```python
from build123d import *

# Parameters (mm, degrees)
ESQUISSE1_W             = 50
ESQUISSE1_H             = 80
BOSS_EXTRU_1_DEPTH      = 2
ENL_V_MAT_EXTRU_1_REACH = 4
ESQUISSE2_R             = 1.75


with BuildPart() as part:
    # Esquisse1 → Boss.-Extru.1 (new body)
    with BuildSketch(Plane(origin=(0, 0, 0), x_dir=(1, 0, 0), z_dir=(0, 1, 0))):
        with Locations((25, 40)):
            Rectangle(ESQUISSE1_W, ESQUISSE1_H)
    extrude(amount=BOSS_EXTRU_1_DEPTH)

    # Esquisse2 → Enlèv. mat.-Extru.1 (cut, up to next)
    with BuildSketch(Plane(origin=(0, 2, 0), x_dir=(1, 0, 0), z_dir=(0, 1, 0)), mode=Mode.PRIVATE) as enl_v_mat_extru_1_sk1:
        with Locations((12.5, 56)):
            Circle(ESQUISSE2_R)
    enl_v_mat_extru_1_tool1 = extrude(enl_v_mat_extru_1_sk1.sketch, amount=-ENL_V_MAT_EXTRU_1_REACH, mode=Mode.PRIVATE) & part.part
    add(enl_v_mat_extru_1_tool1.solids().sort_by_distance((12.5, 2, -56))[0], mode=Mode.SUBTRACT)
    # Esquisse2 → Enlèv. mat.-Extru.1 (cut, up to next)
    with BuildSketch(Plane(origin=(0, 2, 0), x_dir=(1, 0, 0), z_dir=(0, 1, 0)), mode=Mode.PRIVATE) as enl_v_mat_extru_1_sk2:
        with Locations((37.5, 56)):
            Circle(ESQUISSE2_R)
    enl_v_mat_extru_1_tool2 = extrude(enl_v_mat_extru_1_sk2.sketch, amount=-ENL_V_MAT_EXTRU_1_REACH, mode=Mode.PRIVATE) & part.part
    add(enl_v_mat_extru_1_tool2.solids().sort_by_distance((37.5, 2, -56))[0], mode=Mode.SUBTRACT)


solid = part.part
```
Source: CAD feature listing. Evaluate the final solid. Frame: model axes, mm. Give positions to 0.01 mm unless a question says otherwise; leave off trailing zeros. Loops run counter-clockwise (first coordinate to the right, second up) from the corner with the lowest first, then second, coordinate; pieces in that order, holes last. Notation, with made-up numbers: (20, 15.25) -> (47, 15.25) arc R6 cw to (47, 24.25) -> close; hole circle Ø2 at (81, -27). An arc over 180 degrees is marked (long way). Use a Markdown table: item, result. Add a question column.
(1) First-contact query: pin 1 Ø4.5 at (x, z) = (37.5, -56) entering from -Y. Flat tip, straight axial feed; report the tip coordinate or a pass-through.
(2) Ray query, line 1 (X direction, y = 0.65, z = -56); line 2 (Z direction, x = 12.5, y = 1.4). Return the intervals inside material, ascending.
(3) Section query A-A (x = 12.5). Output: boundary loops of the cut face in (y, z).
(4) Section query B-B (z = -56). Output: boundary loops of the cut face in (x, y), then the cut area to 3 significant figures.
(5) Pull-direction query (Z, two-part tool) for faces 1 (the face through (0, 1, -39)), 2 (the face through (25, 1, -80)), 3 (the face through (12.12, 1.01, -54.29)); classes: +Z half, -Z half, draft (parallel to the pull), parting line (faces both ways), or undercut.
Checked values:
| question | item | result |
|---|---|---|
| 1 | pin 1 | y = 0 |
| 2 | line 1 | 0 to 10.75, 14.25 to 35.75, 39.25 to 50 |
| 2 | line 2 | -80 to -57.75, -54.25 to 0 |
| 3 | outline | (0, -80) -> (2, -80) -> (2, -57.75) -> (0, -57.75) -> close; (0, -54.25) -> (2, -54.25) -> (2, 0) -> (0, 0) -> close |
| 4 | outline | (0, 0) -> (10.75, 0) -> (10.75, 2) -> (0, 2) -> close; (14.25, 0) -> (35.75, 0) -> (35.75, 2) -> (14.25, 2) -> close; (39.25, 0) -> (50, 0) -> (50, 2) -> (39.25, 2) -> close |
| 4 | area | 86.0 mm^2 |
| 5 | face 1 | draft |
| 5 | face 2 | -Z half |
| 5 | face 3 | undercut |
